Can you work these out from the drawing? Everything is in mm from the part's minimum corner. A direction names the side the tool comes from. Round coordinates to 2 decimals unless told otherwise and drop trailing zeros. Order: outer loops, then holes, each group sorted by start corner. A loop starts at its lowest first (then second) coordinate and runs counter-clockwise, first axis right, second up. Notation, with made-up numbers: (0.25, 77) - (32.25, 77) arc R33 ccw to (32.25, 111) - close; hole circle Ø5 at (47.25, 18). An arc over 180 degrees is marked (long way). Answer as a JSON object with one key per item and string values.
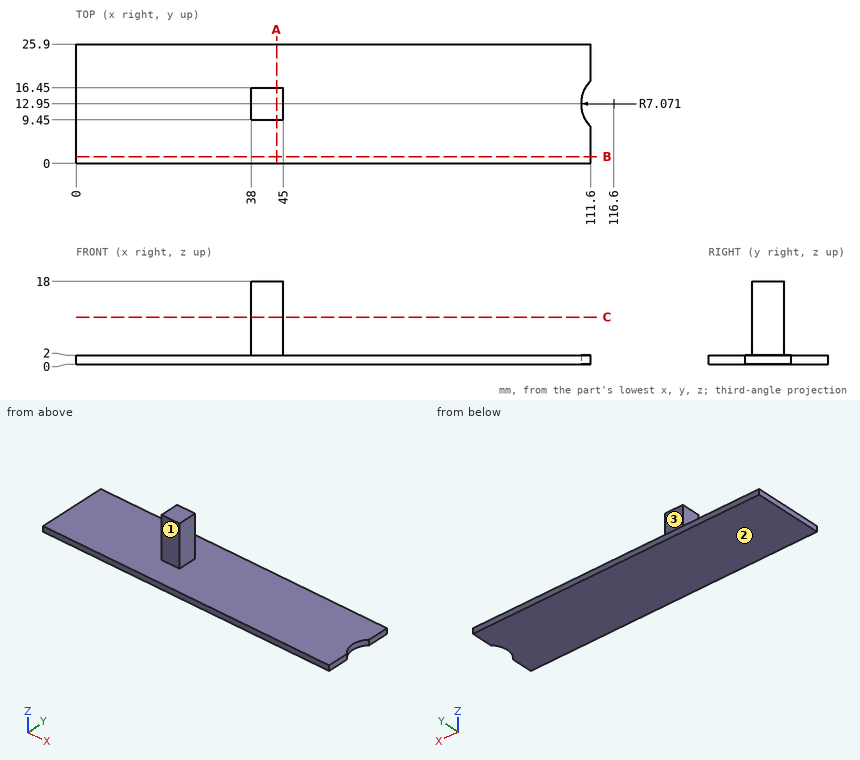
1. If I drill on L1, parallel to Z at x = 76.5, y = 4.25; L2, parallel to X at y = 14, z = 10.75, over which ranges is the centre line in solid material (lowest first)? Write a range as [from, to].
Responses:
{"L1": "[0, 2]", "L2": "[38, 45]"}
2. Imagine slicing it at B-B (y = 1.5). List the corners of the cut face in (x, z) for me.
Responses:
{"outline": "(0, 0) - (111.6, 0) - (111.6, 2) - (0, 2) - close"}
3. Imagine slicing it at C-C (z = 10.25). List the corners of the cut face in (x, y) for me, plus the area to 3 significant figures.
Responses:
{"outline": "(38, 9.45) - (45, 9.45) - (45, 16.45) - (38, 16.45) - close", "area": "49.0 mm2"}
4. Imagine slicing it at A-A (x = 43.5). List the corners of the cut face in (y, z) for me, plus the area to 3 significant figures.
Responses:
{"outline": "(0, 0) - (25.9, 0) - (25.9, 2) - (16.45, 2) - (16.45, 18) - (9.45, 18) - (9.45, 2) - (0, 2) - close", "area": "164 mm2"}
5. For the marked faces 1, 2 and 3, which set-ups out of +Z, -Z, +X, -X, +Y, -Y let a thin tool reach every point of the face, with its end or its side?
Responses:
{"face 1": "+Z, +X, -X, -Y", "face 2": "-Z, +X, -X, +Y, -Y", "face 3": "+Z, +X, -X, +Y"}
6. For P1, Ø7.5, axis at x = 43, z = 13, coming from the -Y side; P2, Ø6, axis at y = 13.5, z = 3.5, coming from the +X side; P3, Ø10, axis at y = 17.5, z = 4, coming from the -X side; P4, Ø5.5, axis at y = 13.5, z = 9, coming from the +X side, each with a flat end and sliding along its axis, tell me the tip position at first contact or that it passes through.
Responses:
{"P1": "y = 9.45", "P2": "x = 110.27", "P3": "x = 0", "P4": "x = 45"}
